The listing builds one solid part. Answer for the finished solid, in the listing's coordinates (mm). Round coordinates to 2 decimals unless told otherwise and drop trailing zeros. Loops run counter-clockwise (first coordinate to the right, second up) from the corner with the lowest first, then second, coordinate; pieces in that order, holes last. Notation, with made-up numbers: M 51,3.25 L 108,3.25 A17 cw 108,7.25 Z; hole C 68,12.5 d8. An arc over 180 degrees is marked long. Answer as a JSON object with one key per item and string values.
Autodesk Inventor part; units mm, degrees
ref_plane "Start Plane" through (0, 0, -4.1685) normal (0, 0, 1) x (1, 0, 0)
ref_plane "End Plane" through (0, 0, 305.0239) normal (0, 0, 1) x (1, 0, 0)
ref_plane "Work Plane4" through (-4.6367, 8.3203, -3.0644) normal (0.1491, -0.2675, -0.9519) x (0.5375, 0.83, -0.1491)
ref_plane "Start Plane" through (0, 0, -4.1685) normal (0, 0, 1) x (1, 0, 0)
ref_plane "End Plane" through (0, 0, 305.0239) normal (0, 0, 1) x (1, 0, 0)
sketch "Sketch" plane through (0, 0, 0) normal (0, 0, 1) x (1, 0, 0)
  circle A0 centre (0, 0) radius 9.525
  dimension "d0" = 19.05
extrude "Body" add sketch "Sketch" along normal up to surface (309.1925 mm away) from surface at -4.1685
sketch "Sketch2" plane through (0, 0, 0) normal (0, 0, 1) x (1, 0, 0)
  line L0 (0, 0) -> (10, 0)
ref_plane "Work Plane3" through (0, 0, 0) normal (0, -1, 0) x (1, 0, 0)
ref_plane "Work Plane4" through (-4.6367, 8.3203, -3.0644) normal (0.1491, -0.2675, -0.9519) x (0.5375, 0.83, -0.1491)
split "Split1" plane through (-4.6367, 8.3203, -3.0644) removes the side toward (0.1491, -0.2675, -0.9519)
ref_plane "Work Plane5" through (-0.6942, 9.4997, 304.378) normal (0.0506, -0.6928, 0.7193) x (0.9985, 0.0204, -0.0506)
split "Split2" plane through (-0.6942, 9.4997, 304.378) removes the side toward (0.0506, -0.6928, 0.7193)
sketch "Sketch3" plane through (0, 0, 0) normal (0, -1, 0) x (1, 0, 0)
  line L0 (-2, -4.1685) -> (12, -4.1685)
  line L1 (-2, 305.0239) -> (12, 305.0239)
  dimension "d7" = 309.1925
equation "\"d0\" = Diam"
equation "\"d1\" = G_L"
equation "\"Diam\" = 19.05"
equation "\"G_L\" = 307.4424"
equation "\"G_OFFSET_START\" = 4.16853"
equation "\"G_OFFSET_END\" = 9.84412"
equation "\"d4\" = -G_OFFSET_START"
equation "\"d5\" = G_OFFSET_END + B_L"
equation "\"B_L\" = 295.17982"
properties part number "ANSI/AISC Rolled Steel - 3/4-12.104, RB" material "Steel, Mild"
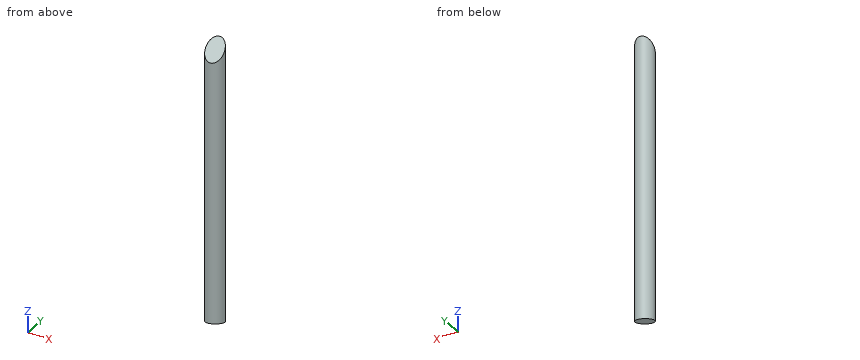
Item 1: The part is cut by section B-B (y = -3). Give the vertices of the cut face in (x, z).
Values follow:
{"outline": "M -9.04,-0.57 L 9.04,2.26 L 9.04,291.65 L -9.04,292.93 Z"}
Item 2: The part is cut by section A-A (z = 193.5). Give the vertices of the cut face in (x, y) (3 decimals).
Values follow:
{"outline": "C 0,0 d19.05"}
Item 3: Straight lines are drawn through the part: line 1 (X direction, y = 0.5, z = 279.5); line 2 (Y direction, x = 1, z = 230); line 3 (Z direction, x = 5.75, y = -5). For each, find the intervals that lie inside material, in ascending order.
Values follow:
{"line 1": "-9.51 to 9.51", "line 2": "-9.47 to 9.47", "line 3": "2.31 to 289.96"}
Item 4: The part is cut by section C-C (x = 2.5). Give the vertices of the cut face in (y, z).
Values follow:
{"outline": "M -9.19,2.97 L 9.19,-2.19 L 9.19,303.86 L -9.19,286.15 Z"}
Item 5: Flat-ended cylindrical pins translate along their axes: P1, Ø2, axis at x = 1.5, y = -7.5, coming from the -Z side; P2, Ø3, axis at y = -4.5, z = 204.5, coming from the -X side; P3, Ø6, axis at x = 6.5, z = 233, coming from the +Y side. Find the tip coordinate at first contact, or state that the pin passes through.
Values follow:
{"P1": "z = 2.02", "P2": "x = -9.04", "P3": "y = 8.86"}
